Could you check a few things on this drawing? It's one solid part, dimensions in mm from its lowest x, y, z. A direction names the side the tool comes from. Give positions to 0.01 mm unless a question says otherwise; leave off trailing zeros. Loops run counter-clockwise (first coordinate to the right, second up) from the corner with the lowest first, then second, coordinate; pieces in that order, holes last.
1. For the marked faces 1 and 2, which set-ups out of +Z, -Z, +X, -X, +Y, -Y let a thin tool reach every point of the face, with its end or its side?
2. Thinking about a two-plate mould opening in Y: for the marked faces 3, 4 and 5, which applies, +Y half, -Y half, draft (parallel to the pull), parting line (faces both ways), or undercut?
3. Imagine slicing it at C-C (z = 7). Count the separate pieces of the cut face and the enclosed holes in it, plus the area to 3 significant figures.
4. Imagine slicing it at D-D (x = 37). List the corners of the cut face in (y, z) for me.
5. I need wall thicknesses on line 1 along X through (y, z) = (36, 4) (1 decimal); line 2 along X through (y, z) = (69, 5.5); line 3 along Y through (x, z) = (8, 5) (1 decimal). Which ranges of each line are inside material? Lowest first, please.
6. Imagine slicing it at B-B (y = 41). List the corners of the cut face in (x, z) for me (1 decimal).
7. Imagine slicing it at A-A (y = 8.76). List the corners of the cut face in (x, z) for me (1 decimal), plus the area to 3 significant figures.
8. For P1, Ø4.5, axis at x = 8.755, y = 68.759, coming from the +Z side; P2, Ø16, axis at x = 38.76, y = 38.76, coming from the -Z side, each with a flat end and sliding along its axis, tell me the tip position at first contact or that it passes through.
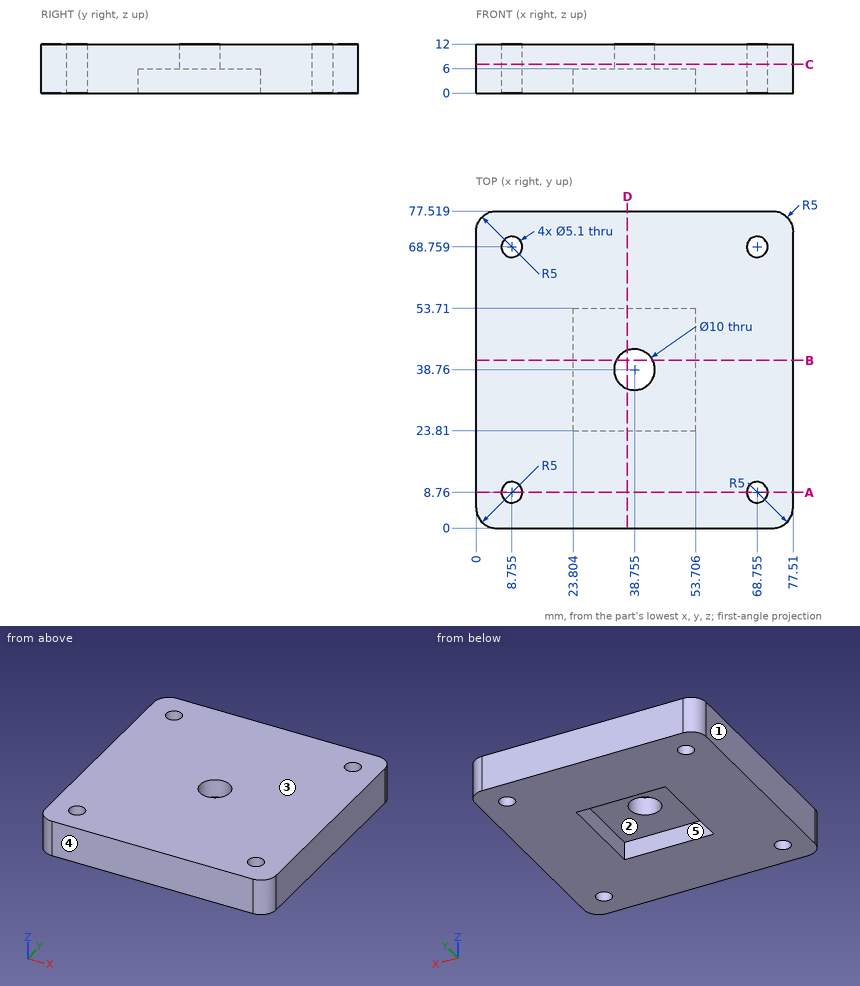
Derived:
1. face 1: +Z, -Z, -X, +Y, -Y
1. face 2: -Z
2. face 3: draft
2. face 4: -Y half
2. face 5: undercut
3. separate pieces: 1
3. enclosed holes: 5
3. area: 5,830 mm2
4. outline: (0, 0) - (23.81, 0) - (23.81, 6) - (34.08, 6) - (34.08, 12) - (0, 12) - close; (43.44, 6) - (53.71, 6) - (53.71, 0) - (77.52, 0) - (77.52, 12) - (43.44, 12) - close
5. line 1: x = 0 to 23.8, 53.7 to 77.5
5. line 2: x = 0 to 6.22, 11.29 to 66.22, 71.29 to 77.51
5. line 3: y = 0 to 6.3, 11.2 to 66.3, 71.2 to 77.5
6. outline: (0, 0) - (23.8, 0) - (23.8, 6) - (34.3, 6) - (34.3, 12) - (0, 12) - close; (43.2, 6) - (53.7, 6) - (53.7, 0) - (77.5, 0) - (77.5, 12) - (43.2, 12) - close
7. outline: (0, 0) - (6.2, 0) - (6.2, 12) - (0, 12) - close; (11.3, 0) - (66.2, 0) - (66.2, 12) - (11.3, 12) - close; (71.3, 0) - (77.5, 0) - (77.5, 12) - (71.3, 12) - close
7. area: 808 mm2
8. P1: passes through
8. P2: stops at z = 6
